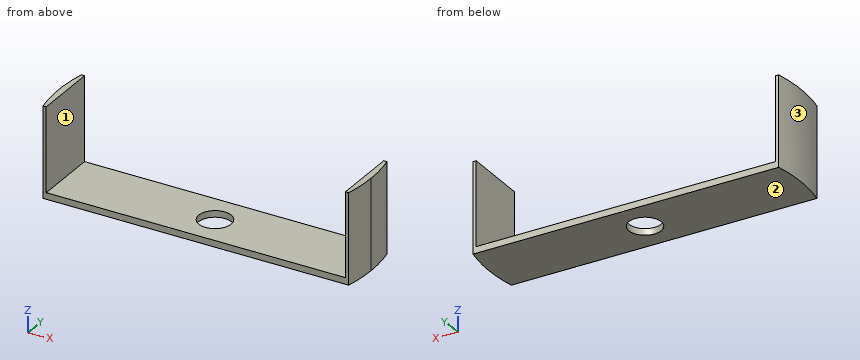
from build123d import *

# Parameters (mm, degrees)
F1_DEPTH = 56
F2_W     = 184.809428
F2_H     = 40
F2_R     = 10
F3_DEPTH = 52
F4_DEPTH = 60


with BuildPart() as f1:
    # F0 (on Top) → F1 (new body)
    with BuildSketch(Plane.XY):
        with BuildLine():
            ThreePointArc((94.404714, -20), (95.974749, -10.054728), (96.5, 0))
            ThreePointArc((96.5, 0), (95.974749, 10.054728), (94.404714, 20))
            Line((94.404714, 20), (0, 20))
            Line((0, 20), (-94.404714, 20))
            ThreePointArc((-94.404714, 20), (-96.5, 0), (-94.404714, -20))
            Line((-94.404714, -20), (0, -20))
            Line((0, -20), (94.404714, -20))
        make_face()
    extrude(amount=F1_DEPTH)

    # F2 (on face) → F3 (cut)
    with BuildSketch(Plane.XY.offset(56)):
        Rectangle(F2_W, F2_H)
        Circle(F2_R, mode=Mode.SUBTRACT)
    extrude(amount=-F3_DEPTH, mode=Mode.SUBTRACT)

    # F2 (on face) → F4 (cut)
    with BuildSketch(Plane.XY.offset(56)):
        Circle(F2_R)
    extrude(amount=-F4_DEPTH, mode=Mode.SUBTRACT)


solid = f1.part
Part model, mm, in its own coordinate system. Face numbers are marked on the shaded views. Coordinates: 2 decimals unless noted, no trailing zeros. Loops run counter-clockwise (first coordinate to the right, second up) from the corner with the lowest first, then second, coordinate; pieces in that order, holes last. Notation, with made-up numbers: (43, 17) -> (95, 17) arc R22 cw to (95, 43) -> close; hole circle Ø8 at (-21, -9). An arc over 180 degrees is marked (long way). Use a Markdown table: item, result. Add a question column.
Item 1: Band-saw the part on A-A on z = 9. Write the cut outline in (x, y), plus the area to 3 significant figures.
Item 2: Pull direction X, two halves, no side cores. Call the marked faces 1, 2 and 3: +X half, -X half, draft (parallel to the pull), parting line (faces both ways), or undercut.
Item 3: Band-saw the part on D-D on y = 3. Write the cut outline in (x, z), plus the area to 3 significant figures.
Item 4: Band-saw the part on B-B on x = 0. Write the cut outline in (y, z), plus the area to 3 significant figures.
Item 5: Probe probe 1 along X at (y, z) = (-1, 51.5); probe 2 along Y at (x, z) = (0, 1.3); probe 3 along Z at (x, y) = (-15, 2.5). List the from-to ranges inside material, lowest first.
Item 6: Band-saw the part on C-C on y = -7.5. Write the cut outline in (x, z), plus the area to 3 significant figures.
Item 7: Flat gauge pins, fed straight in: P1, Ø16, axis at x = 0, y = 0, coming from the +Z side; P2, Ø8, axis at y = -12, z = 43, coming from the -X side; P3, Ø1, axis at y = 15.5, z = 35.5, coming from the -X side; P4, Ø2, axis at x = 13, y = 12.5, coming from the +Z side. Where does each tip first touch, or does it go through?
Geometry says:
| question | item | result |
|---|---|---|
| 1 | outline | (-94.4, -20) -> (-92.4, -20) -> (-92.4, 20) -> (-94.4, 20) arc R96.5 ccw to start; (92.4, -20) -> (94.4, -20) arc R96.5 ccw to (96.5, 0) arc R96.5 ccw to (94.4, 20) -> (92.4, 20) -> close |
| 1 | area | 272 mm² |
| 2 | face 1 | undercut |
| 2 | face 2 | draft |
| 2 | face 3 | -X half |
| 3 | outline | (-96.45, 0) -> (-9.54, 0) -> (-9.54, 4) -> (-92.4, 4) -> (-92.4, 56) -> (-96.45, 56) -> close; (9.54, 0) -> (96.45, 0) -> (96.45, 56) -> (92.4, 56) -> (92.4, 4) -> (9.54, 4) -> close |
| 3 | area | 1,120 mm² |
| 4 | outline | (-20, 0) -> (-10, 0) -> (-10, 4) -> (-20, 4) -> close; (10, 0) -> (20, 0) -> (20, 4) -> (10, 4) -> close |
| 4 | area | 80.0 mm² |
| 5 | probe 1 | -96.49 to -92.4, 92.4 to 96.49 |
| 5 | probe 2 | -20 to -10, 10 to 20 |
| 5 | probe 3 | 0 to 4 |
| 6 | outline | (-96.21, 0) -> (-6.61, 0) -> (-6.61, 4) -> (-92.4, 4) -> (-92.4, 56) -> (-96.21, 56) -> close; (6.61, 0) -> (96.21, 0) -> (96.21, 56) -> (92.4, 56) -> (92.4, 4) -> (6.61, 4) -> close |
| 6 | area | 1,110 mm² |
| 7 | P1 | through |
| 7 | P2 | x = -96.17 |
| 7 | P3 | x = -95.33 |
| 7 | P4 | z = 4 |
